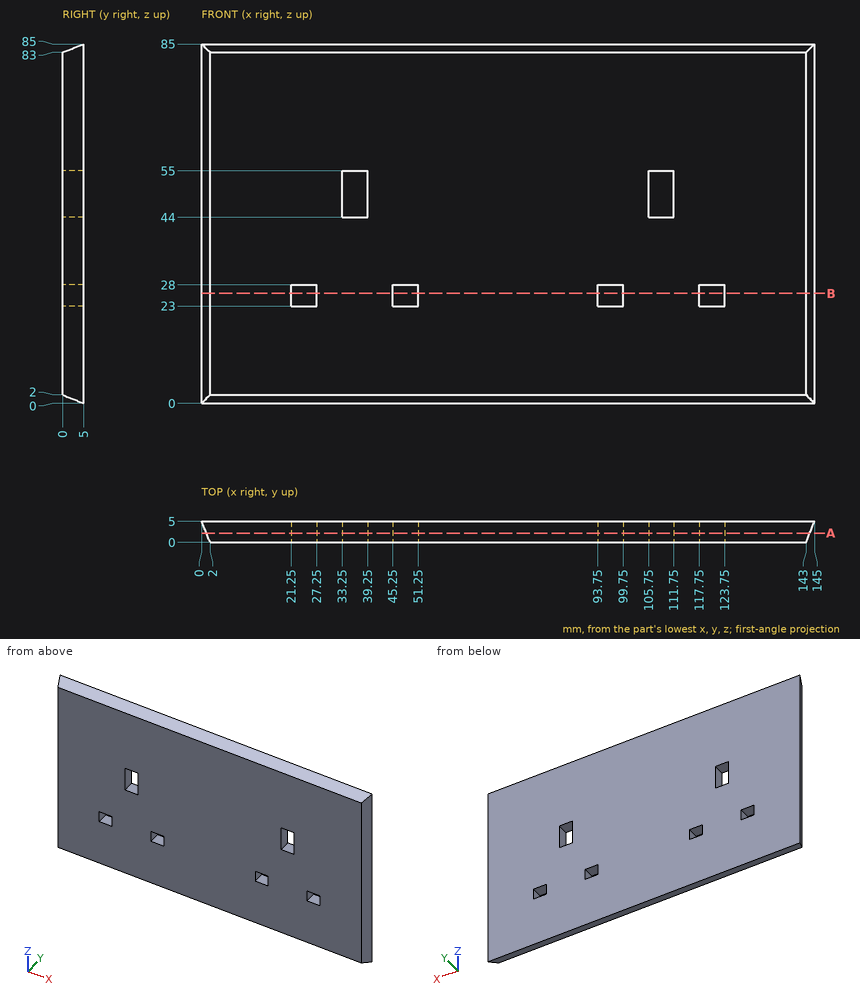
Verification items for this drawing (mm, ordinates from the low corner). Give positions to 0.01 mm unless a question says otherwise; leave off trailing zeros. Loops run counter-clockwise (first coordinate to the right, second up) from the corner with the lowest first, then second, coordinate; pieces in that order, holes last.
(1) Depth check by flat-ended pin: pin 1 Ø1.5 at (x, y) = (109, 2) entering from -Z; pin 2 Ø2.5 at (x, y) = (121.5, 2.5) entering from -Z; pin 3 Ø1.5 at (y, z) = (2, 47.5) entering from -X. Enter the tip coordinate at first touch or a pass-through.
From the geometry:
pin 1: stops at z = 0.9
pin 2: stops at z = 0.5
pin 3: stops at x = 0.9
(2) Section check A-A on y = 2.2. Record the cut outline in (x, z), then the cut area to 3 significant figures.
From the geometry:
outline: (1.12, 1.12) - (143.88, 1.12) - (143.88, 83.88) - (1.12, 83.88) - close; hole (21.25, 23) - (27.25, 23) - (27.25, 28) - (21.25, 28) - close; hole (33.25, 44) - (39.25, 44) - (39.25, 55) - (33.25, 55) - close; hole (45.25, 23) - (51.25, 23) - (51.25, 28) - (45.25, 28) - close; hole (93.75, 23) - (99.75, 23) - (99.75, 28) - (93.75, 28) - close; hole (105.75, 44) - (111.75, 44) - (111.75, 55) - (105.75, 55) - close; hole (117.75, 23) - (123.75, 23) - (123.75, 28) - (117.75, 28) - close
area: 11,600 mm2
(3) Thickness scan on L1, parallel to X at y = 2.75, z = 49.5; L2, parallel to Z at x = 96.5, y = 2.95; L3, parallel to Z at x = 36.5, y = 1.7. Record the ranges inside material, lowest first.
From the geometry:
L1: x = 0.9 to 33.25, 39.25 to 105.75, 111.75 to 144.1
L2: z = 0.82 to 23, 28 to 84.18
L3: z = 1.32 to 44, 55 to 83.68
(4) Section check B-B on z = 26. Count the separate pieces of the cut face and the enclosed holes in it, then the cut area to 3 significant figures.
From the geometry:
separate pieces: 5
enclosed holes: 0
area: 595 mm2
